```python
from build123d import *

# Parameters (mm, degrees)
SKETCH1_W           = 20
SKETCH1_H           = 13
SKETCH1_R           = 3.25
SKETCH1_H_2         = 34
BOSS_EXTRUDE1_DEPTH = 32.8
BOSS_EXTRUDE2_START = 32.8
SKETCH1_3_W         = 20
SKETCH1_3_H         = 34
BOSS_EXTRUDE2_DEPTH = 10.5
SKETCH2_OUTSIDE_W   = 60.63
SKETCH2_OUTSIDE_H   = 77.33
SKETCH2_OUTSIDE_R   = 6.1
SKETCH2_OUTSIDE_R_2 = 3.25
CUT_EXTRUDE1_DEPTH  = 295.275


with BuildPart() as part:
    # Sketch1 → Boss-Extrude1 (new body)
    # profile 1 of 3: a face of its own
    with BuildSketch(Plane.XY):
        with Locations((-285.275, 23.5)):
            Rectangle(SKETCH1_W, SKETCH1_H)
        with Locations((-285.275, 23)):
            Circle(SKETCH1_R, mode=Mode.SUBTRACT)
    # profile 2 of 3: a face of its own
    with BuildSketch(Plane.XY):
        with Locations((-285.275, 0)):
            Rectangle(SKETCH1_W, SKETCH1_H_2)
    # profile 3 of 3: a face of its own
    with BuildSketch(Plane.XY):
        with Locations((-285.275, -23.5)):
            Rectangle(SKETCH1_W, SKETCH1_H)
        with Locations((-285.275, -23)):
            Circle(SKETCH1_R, mode=Mode.SUBTRACT)
    extrude(amount=BOSS_EXTRUDE1_DEPTH)

    # Sketch1<3> → Boss-Extrude2 (add)
    with BuildSketch(Plane.XY.offset(BOSS_EXTRUDE2_START)):
        with Locations((-285.275, 0)):
            Rectangle(SKETCH1_3_W, SKETCH1_3_H)
    extrude(amount=BOSS_EXTRUDE2_DEPTH)

    # Sketch2 outside → Cut-Extrude1 (cut)
    # profile 1 of 6: a face of its own
    with BuildSketch(Plane(origin=(0, 0, 0), x_dir=(0, 0, -1), z_dir=(1, 0, 0))):
        with Locations((-21.65, 0)):
            Rectangle(SKETCH2_OUTSIDE_W, SKETCH2_OUTSIDE_H)
        Polygon((0, -30), (0, 30), (-32.8, 30), (-32.8, 17), (-43.3, 17), (-43.3, -17), (-32.8, -17), (-32.8, -30), align=None, mode=Mode.SUBTRACT)
    # profile 2 of 6: a face of its own
    with BuildSketch(Plane(origin=(0, 0, 0), x_dir=(0, 0, -1), z_dir=(1, 0, 0))):
        with Locations(Location((-25.4, 0, 0), (0, 0, 180))):
            Circle(SKETCH2_OUTSIDE_R)
    # profile 3 of 6: a face of its own
    with BuildSketch(Plane(origin=(0, 0, 0), x_dir=(0, 0, -1), z_dir=(1, 0, 0))):
        with Locations(Location((-7.9, -22.5, 0), (0, 0, 180))):
            Circle(SKETCH2_OUTSIDE_R_2)
    # profile 4 of 6: a face of its own
    with BuildSketch(Plane(origin=(0, 0, 0), x_dir=(0, 0, -1), z_dir=(1, 0, 0))):
        with Locations(Location((-24.9, -22.5, 0), (0, 0, 180))):
            Circle(SKETCH2_OUTSIDE_R_2)
    # profile 5 of 6: a face of its own
    with BuildSketch(Plane(origin=(0, 0, 0), x_dir=(0, 0, -1), z_dir=(1, 0, 0))):
        with Locations(Location((-24.9, 22.5, 0), (0, 0, 180))):
            Circle(SKETCH2_OUTSIDE_R_2)
    # profile 6 of 6: a face of its own
    with BuildSketch(Plane(origin=(0, 0, 0), x_dir=(0, 0, -1), z_dir=(1, 0, 0))):
        with Locations(Location((-7.9, 22.5, 0), (0, 0, 180))):
            Circle(SKETCH2_OUTSIDE_R_2)
    extrude(amount=-CUT_EXTRUDE1_DEPTH, mode=Mode.SUBTRACT)


solid = part.part
```
The model under review builds one solid part; all positions refer to its coordinate system, in mm. A direction names the side the tool comes from. Coordinates: 2 decimals unless noted, no trailing zeros. Write each loop counter-clockwise with the first axis right and the second up, starting at its lowest first coordinate (ties: lowest second). Pieces come first, ordered by that corner, then holes. Notation, with made-up numbers: (6.25, 29.5) - (50.25, 29.5) arc R27 ccw to (50.25, 50.5) - close; hole circle Ø11 at (79, -16.75). An arc over 180 degrees is marked (long way). Answer in a Markdown table with one row per item. Add a question column.
Q1. For faces 1 (the face through (-285, -17, 38)), 2 (the face through (-285.135, -0.268, 19.306)), 3 (the face through (-285, 17, 38)), list the 3-axis set-ups (+Z, -Z, +X, -X, +Y, -Y) from which the entire face can be reached by the end or side of a thin tool; tool diameter is ignored.
Q2. Consider section D-D on y = -24. Give the boundary of the cut face in (x, z) (3 decimals), then the cut area to 3 significant figures.
Q3. Consider section A-A on y = 0. Give the boundary of the cut face in (x, z) (3 decimals), then the cut area to 3 significant figures.
Q4. Consider section B-B on z = 13. Give the boundary of the cut face in (x, y) (3 decimals), then the cut area to 3 significant figures.
Q5. Consider section C-C on x = -291.75. Give the boundary of the cut face in (y, z).
Q6. Draft analysis for pull direction Z (two halves, no side actions). For faces 4 (the face through (-295.275, 0, 17)), 5 (the face through (-285, 0, 43.3)), 6 (the face through (-285.135, 19.278, 24.477)), 7 (the face through (-285.135, -19.327, 7.195)), state which applies: +Z half, -Z half, draft (parallel to the pull), parting line (faces both ways), or undercut.
Q7. Clearance check with flat-ended pins moving along their axes: pin 1 (6 mm diameter, centred on y = 22.5, z = 7.9, fed in from +X); pin 2 (11.5 mm diameter, centred on x = -284.5, z = 40.5, fed in from -Y); pin 3 (6 mm diameter, centred on x = -280, y = 22, fed in from +Z). State where each tip first meets the part, or that it passes through.
Q8. To check wall thickness, follow line 1 along Z through (x, y) = (-290, -22.5); line 2 along Y through (x, z) = (-282.25, 7.9); line 3 along Y through (x, z) = (-293.5, 10.5). State the ranges of each line that lie inside material, in increasing order. Write a range as from..to.
Answers below:
| question | item | result |
|---|---|---|
| 1 | face 1 | +Z, +X, -X, -Y |
| 1 | face 2 | +X, -X |
| 1 | face 3 | +Z, +X, -X, +Y |
| 2 | outline | (-295.275, 0) - (-288.367, 0) - (-288.367, 5.017) - (-295.275, 5.017) - close; (-295.275, 10.783) - (-288.367, 10.783) - (-288.367, 22.017) - (-295.275, 22.017) - close; (-295.275, 27.783) - (-288.367, 27.783) - (-288.367, 32.8) - (-295.275, 32.8) - close; (-282.183, 0) - (-275.275, 0) - (-275.275, 5.017) - (-282.183, 5.017) - close; (-282.183, 10.783) - (-275.275, 10.783) - (-275.275, 22.017) - (-282.183, 22.017) - close; (-282.183, 27.783) - (-275.275, 27.783) - (-275.275, 32.8) - (-282.183, 32.8) - close |
| 2 | area | 294 mm² |
| 3 | outline | (-295.275, 0) - (-275.275, 0) - (-275.275, 19.3) - (-295.275, 19.3) - close; (-295.275, 31.5) - (-275.275, 31.5) - (-275.275, 43.3) - (-295.275, 43.3) - close |
| 3 | area | 622 mm² |
| 4 | outline | (-295.275, -30) - (-275.275, -30) - (-275.275, 30) - (-295.275, 30) - close; hole circle Ø6.5 at (-285.275, -23); hole circle Ø6.5 at (-285.275, 23) |
| 4 | area | 1,130 mm² |
| 5 | outline | (-30, 0) - (30, 0) - (30, 32.8) - (17, 32.8) - (17, 43.3) - (-17, 43.3) - (-17, 32.8) - (-30, 32.8) - close; hole circle Ø6.5 at (-22.5, 7.9); hole circle Ø6.5 at (-22.5, 24.9); hole circle Ø12.2 at (0, 25.4); hole circle Ø6.5 at (22.5, 7.9); hole circle Ø6.5 at (22.5, 24.9) |
| 6 | face 4 | draft |
| 6 | face 5 | +Z half |
| 6 | face 6 | undercut |
| 6 | face 7 | undercut |
| 7 | pin 1 | through |
| 7 | pin 2 | y = -17 |
| 7 | pin 3 | z = 32.8 |
| 8 | line 1 | 0..4.65, 11.15..21.65, 28.15..32.8 |
| 8 | line 2 | -30..-25.75, -19.25..19.25, 25.75..30 |
| 8 | line 3 | -30..-24.45, -20.55..20.55, 24.45..30 |
